Source: CAD feature listing. Evaluate the final solid. Frame: model axes, mm. A direction names the side the tool comes from. Round coordinates to 2 decimals unless told otherwise and drop trailing zeros. Loops run counter-clockwise (first coordinate to the right, second up) from the corner with the lowest first, then second, coordinate; pieces in that order, holes last.
Item 1: First-contact query: P1, Ø3.5, axis at y = 0, z = 0, coming from the -X side; P2, Ø3, axis at y = -0.5, z = 0.5, coming from the +X side; P3, Ø2.5, axis at y = 0.5, z = 0, coming from the +X side; P4, Ø1.5, axis at x = 6, z = 9, coming from the -Y side. Flat tips, straight axial feed; report the tip coordinate or a pass-through.
Item 2: Pull-direction query (Z, two-part tool) for faces 6 (the conical face through (-2.07, 3.6, 10.41)), 7 (the flat face through (-3.48, -1.97, 7.54)), 8 (the cylindrical face through (14.9, -0.1, -4.9)), 9 (the flat face through (4.1, 0, 1)); classes: released by +Z, released by -Z, zero draft, split by the parting line, or undercut.
Item 3: Ray query, L1, parallel to Y at x = 1.3, z = 0; L2, parallel to X at y = 1.75, z = 2.25; L3, parallel to Z at x = 2.7, y = 0. Return the intervals inside material, ascending.
Item 4: Section query B-B on z = 4.25. Give the number of separate pieces and of enclosed holes in the cut face, then the cut area to 3 significant figures.
Item 5: Access query for faces 1 (the conical face through (2.07, -3.6, 10.41)), 2 (the cylindrical face through (-0.167, -3.796, 11.297)), 3 (the flat face through (15, -3.9, 0)), 4 (the conical face through (-4.15, 0.01, 10.413)), 5 (the conical face through (4.148, -0.01, 4.585)). Directions: +Z, -Z, +X, -X, +Y, -Y. A direction counts if a zero-diameter tool reaches every point of the face in a straight line with its end or side. Return the directions, or none.
Item 6: Section query A-A on x = 9. Return loops of the section in (y, z), then the cut area to 3 significant figures.
```python
from build123d import *

# Parameters (mm, degrees)
CUT_EXTRUDE1_DEPTH = 1.2
SKETCH5_W          = 14
SKETCH5_H          = 0.65
SKETCH7_W          = 16
SKETCH7_H          = 16
CUT_EXTRUDE2_DEPTH = 7.055555556


with BuildPart() as part:
    # Sketch1 → Revolve1 (revolve)
    with BuildSketch(Plane.XY):
        with BuildLine():
            Line((0, 2.8), (2.8, 2.8))
            Line((2.8, 2.8), (4, 4))
            Line((4, 4), (12.457142857, 4))
            Line((12.457142857, 4), (13.2, 3.800952028))
            Line((13.2, 3.800952028), (13.2, 3.693772352))
            Line((13.2, 3.693772352), (13.458578644, 3.693772352))
            Line((13.458578644, 3.693772352), (13.6, 3.552350995))
            Line((13.6, 3.552350995), (13.6, 2.5))
            Line((13.6, 2.5), (14.13, 2.5))
            ThreePointArc((14.13, 2.5), (14.391629509, 2.608370491), (14.5, 2.87))
            Line((14.5, 2.87), (14.5, 5.9))
            Line((14.5, 5.9), (14.897402943, 5.9))
            ThreePointArc((14.897402943, 5.9), (15.025960465, 5.853208889), (15.094364494, 5.734729636))
            Line((15.094364494, 5.734729636), (15.7, 2.3))
            Line((15.7, 2.3), (15.7, 0))
            Line((15.7, 0), (-2.8, 0))
            ThreePointArc((-2.8, 0), (-1.979898987, 1.979898987), (0, 2.8))
        make_face()
    revolve(axis=Axis((15.7, 0, 0), (-1, 0, 0)))

    # Sketch2 → Revolve2 (revolve)
    with BuildSketch(Plane(origin=(0, 0, 0), x_dir=(0, 0, -1), z_dir=(1, 0, 0))):
        Polygon((-11.5, 0), (-11.5, 3.8), (-11.1, 3.8), (-11, 3.7), (-10.9, 3.8), (-10.5, 3.8), (-10.5, 4), (-10.130495828, 4.64), (-4.869504172, 4.64), (-4.5, 4), (-4.5, 3), (-2.8, 3), (-2.6, 2.8), (0, 2.8), (0, 0), align=None)
    revolve(axis=Axis((0, 0, 0), (0, 0, 1)))

    # Sketch3 → Revolve3 (revolve)
    with BuildSketch(Plane(origin=(0, 0, 0), x_dir=(0, 0, -1), z_dir=(1, 0, 0))):
        Polygon((-14, 0), (-14, 1.1935), (-13.6935, 1.5), (-11.5, 1.5), (-11.5, 0), align=None)
    revolve(axis=Axis((0, 0, 11.5), (0, 0, 1)))

    # Sketch4 → Cut-Extrude1 (cut)
    with BuildSketch(Plane(origin=(15.7, 0, 0), x_dir=(0, 0, -1), z_dir=(1, 0, 0))):
        Polygon((-9.8, -5.658032638), (0, -11.316065276), (9.8, -5.658032638), (9.8, 5.658032638), (0, 11.316065276), (-9.8, 5.658032638), align=None)
        with BuildLine():
            Line((-1, -3.9), (1, -3.9))
            ThreePointArc((1, -3.9), (4.9, 0), (1, 3.9))
            Line((1, 3.9), (-1, 3.9))
            ThreePointArc((-1, 3.9), (-4.9, 0), (-1, -3.9))
        make_face(mode=Mode.SUBTRACT)
    extrude(amount=-CUT_EXTRUDE1_DEPTH, mode=Mode.SUBTRACT)

    # Sketch5 → Cut-Revolve1 (revolve, cut)
    with BuildSketch(Plane(origin=(0, 0, 0), x_dir=(0, 0, -1), z_dir=(1, 0, 0))):
        with Locations((-7, 0.325)):
            Rectangle(SKETCH5_W, SKETCH5_H)
    revolve(axis=Axis((0, 0, 0), (0, 0, 1)), mode=Mode.SUBTRACT)

    # Sketch6 → Cut-Revolve2 (revolve, cut)
    with BuildSketch(Plane(origin=(0, 0, 0), x_dir=(1, 0, 0), z_dir=(0, 1, 0))):
        with BuildLine():
            Line((0, 0.65), (4.1, 0.65))
            Line((4.1, 0.65), (4.1, 2))
            Line((4.1, 2), (15.4, 2))
            ThreePointArc((15.4, 2), (15.612132034, 2.087867966), (15.7, 2.3))
            Line((15.7, 2.3), (15.7, 0))
            Line((15.7, 0), (-0.65, 0))
            ThreePointArc((-0.65, 0), (-0.459619408, 0.459619408), (0, 0.65))
        make_face()
    revolve(axis=Axis((15.7, 0, 0), (-1, 0, 0)), mode=Mode.SUBTRACT)

    # Sketch7 → Cut-Extrude2 (cut)
    with BuildSketch(Plane.XY.offset(11.5)):
        Rectangle(SKETCH7_W, SKETCH7_H)
        Polygon((-4.618802154, 0), (-2.309401077, -4), (2.309401077, -4), (4.618802154, 0), (2.309401077, 4), (-2.309401077, 4), align=None, mode=Mode.SUBTRACT)
    extrude(amount=-CUT_EXTRUDE2_DEPTH, mode=Mode.SUBTRACT)


solid = part.part
```
Data:
1. P1: stops at x = -2.8
1. P2: stops at x = 15.69
1. P3: stops at x = 4.1
1. P4: passes through
2. face 6: released by +Z
2. face 7: zero draft
2. face 8: released by -Z
2. face 9: undercut
3. L1: y = -2.8 to -0.65, 0.65 to 2.8
3. L2: x = -2.19 to 2.19, 2.85 to 13.6, 14.5 to 15.6
3. L3: z = -2.8 to -0.65, 0.65 to 11.5
4. separate pieces: 2
4. enclosed holes: 1
4. area: 30.5 mm2
5. face 1: +Z, +X, -Y
5. face 2: +Z
5. face 3: +Z, -Z, +X, -Y
5. face 4: +Z, -X
5. face 5: none
6. outline: circle Ø8 at (0, 0); hole circle Ø4 at (0, 0)
6. area: 37.7 mm2
